Source: three-view drawing plus pictorial views. Frame: mm from the lowest corner of the part. A direction names the side the tool comes from. Give positions to 0.01 mm unless a question says otherwise; leave off trailing zeros. Order: outer loops, then holes, each group sorted by start corner. A loop starts at its lowest first (then second) coordinate and runs counter-clockwise, first axis right, second up. Notation, with made-up numbers: (80.25, 14) -> (137.25, 14) arc R21 cw to (137.25, 30) -> close; hole circle Ø6 at (-17, 15). An arc over 180 degrees is marked (long way). Answer in a Markdown table with one row per item. Add a question column.
Q1. Cut plane C-C on x = 3.78. Return the cut outline in (y, z).
Q2. Set-up query: the marked faces 1, 2, 3 and 4. Return all of +Z, -Z, +X, -X, +Y, -Y with unobstructed straight access to the full face (end or side cutting, diameter ignored); none if empty.
Q3. Line query: line 1 along X through (y, z) = (1.5, 26.68); line 2 along X through (y, z) = (3.15, 17); line 3 along Y through (x, z) = (10.5, 9). Output: solid intervals per line, ascending. Write a range as from..to.
Q4. Cut plane D-D on x = 21. Return the cut outline in (y, z).
Q5. Contact query for flat-ended pins moving along their axis: P1, Ø1.6, axis at x = 36.5, z = 14.5, coming from the -Y side; P2, Ø1.2, axis at x = 31, y = 3.5, coming from the +Z side (3 decimals); P3, Ø2.5, axis at x = 31.78, z = 3.83, coming from the -Y side; P4, Ø1, axis at x = 23, z = 12, coming from the +Y side. Output: stop coordinate, or through.
Q6. Cut plane B-B on z = 3.83. Return the cut outline in (x, y), and give its area (3 significant figures).
Q7. Cut plane A-A on x = 31.78. Return the cut outline in (y, z) (3 decimals), and give its area (3 significant figures).
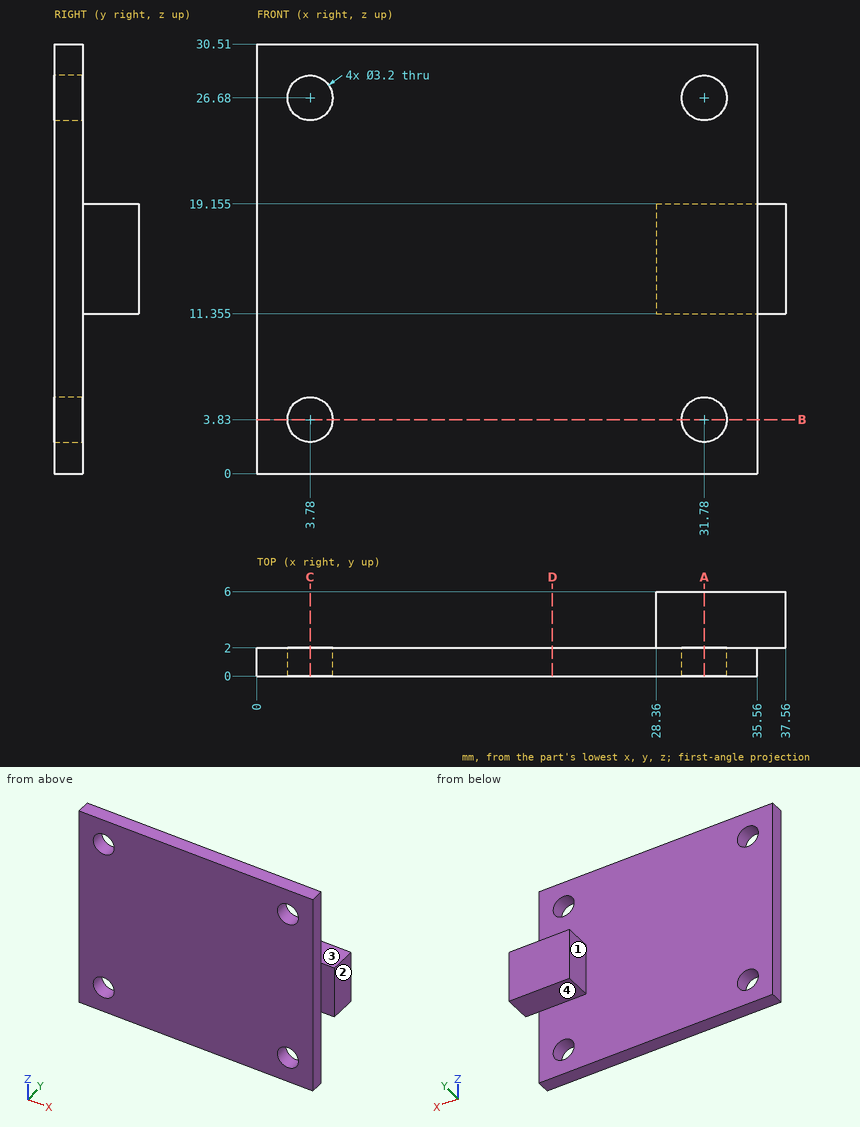
Completed:
| question | item | result |
|---|---|---|
| 1 | outline | (0, 0) -> (2, 0) -> (2, 2.23) -> (0, 2.23) -> close; (0, 5.43) -> (2, 5.43) -> (2, 25.08) -> (0, 25.08) -> close; (0, 28.28) -> (2, 28.28) -> (2, 30.51) -> (0, 30.51) -> close |
| 2 | face 1 | +Z, -Z, -X, +Y |
| 2 | face 2 | +Z, -Z, +X, +Y, -Y |
| 2 | face 3 | +Z, +X, -X, +Y |
| 2 | face 4 | -Z, +X, -X, +Y |
| 3 | line 1 | x = 0..2.18, 5.38..30.18, 33.38..35.56 |
| 3 | line 2 | x = 28.36..37.56 |
| 3 | line 3 | y = 0..2 |
| 4 | outline | (0, 0) -> (2, 0) -> (2, 30.51) -> (0, 30.51) -> close |
| 5 | P1 | stops at y = 2 |
| 5 | P2 | stops at z = 19.155 |
| 5 | P3 | passes through |
| 5 | P4 | stops at y = 2 |
| 6 | outline | (0, 0) -> (2.18, 0) -> (2.18, 2) -> (0, 2) -> close; (5.38, 0) -> (30.18, 0) -> (30.18, 2) -> (5.38, 2) -> close; (33.38, 0) -> (35.56, 0) -> (35.56, 2) -> (33.38, 2) -> close |
| 6 | area | 58.3 mm² |
| 7 | outline | (0, 0) -> (2, 0) -> (2, 2.23) -> (0, 2.23) -> close; (0, 5.43) -> (2, 5.43) -> (2, 11.355) -> (6, 11.355) -> (6, 19.155) -> (2, 19.155) -> (2, 25.08) -> (0, 25.08) -> close; (0, 28.28) -> (2, 28.28) -> (2, 30.51) -> (0, 30.51) -> close |
| 7 | area | 79.4 mm² |
